For this review, take the finished solid that the model builds, in its own axes (mm). A direction names the side the tool comes from. Coordinates: 2 decimals unless noted, no trailing zeros. Loops run counter-clockwise (first coordinate to the right, second up) from the corner with the lowest first, then second, coordinate; pieces in that order, holes last. Notation, with made-up numbers: M 66,61 L 107,61 A17 cw 107,83 Z; hole C 30.5,-34 d9. An arc over 180 degrees is marked long. Use one line per item in the form item = value.
```python
from build123d import *

# Parameters (mm, degrees)
F0_W     = 80
F0_H     = 40
F1_DEPTH = 10
F2_W     = 74
F2_H     = 26
F3_DEPTH = 5
F4_W     = 4
F4_H     = 4
F5_DEPTH = 25.4
F6_W     = 4
F6_H     = 4
F7_DEPTH = 50.8


with BuildPart() as f1:
    # F0 (on Front) → F1 (new body)
    with BuildSketch(Plane.XZ):
        with Locations((40, 20)):
            Rectangle(F0_W, F0_H)
    extrude(amount=F1_DEPTH)

    # F2 (on face) → F3 (cut)
    with BuildSketch(Plane.XZ.offset(10)):
        with Locations((40, 20)):
            Rectangle(F2_W, F2_H)
    extrude(amount=-F3_DEPTH, mode=Mode.SUBTRACT)

    # F4 (on face) → F5 (cut)
    with BuildSketch(Plane.XZ.offset(10)):
        with Locations((6, 38)):
            Rectangle(F4_W, F4_H)
        with Locations((74, 38)):
            Rectangle(F4_W, F4_H)
        with Locations((74, 2)):
            Rectangle(F4_W, F4_H)
        with Locations((6, 2)):
            Rectangle(F4_W, F4_H)
    extrude(amount=-F5_DEPTH, mode=Mode.SUBTRACT)

    # F6 (on face) → F7 (cut)
    with BuildSketch(Plane.XY.offset(40)):
        with Locations((6, -2)):
            Rectangle(F6_W, F6_H)
        with Locations((74, -2)):
            Rectangle(F6_W, F6_H)
    extrude(amount=-F7_DEPTH, mode=Mode.SUBTRACT)


solid = f1.part
```
1. Draft analysis for pull direction Z (two halves, no side actions). For faces 1 (the face through (39, -8, 7)), 2 (the face through (74, -7, 4)), 3 (the face through (6, -4, 20)), 4 (the face through (39, -8, 33)), state which applies: +Z half, -Z half, draft (parallel to the pull), parting line (faces both ways), or undercut.
Computed values:
face_1 = undercut
face_2 = -Z half
face_3 = draft
face_4 = undercut
2. For pin 1 Ø1.2 at (x, y) = (74.5, -7) entering from -Z; pin 2 Ø1 at (x, z) = (13, 13.5) entering from -Y; pin 3 Ø1.2 at (x, z) = (5.5, 26.5) entering from +Y, all flat-tipped, find the tip position at first contact; note any pin that passes through.
Computed values:
pin_1 = 4
pin_2 = -5
pin_3 = -4
3. Consider section D-D on y = -8.5. Write out the cut boundary in (x, z).
Computed values:
outline = M 0,0 L 4,0 L 4,4 L 8,4 L 8,0 L 72,0 L 72,4 L 76,4 L 76,0 L 80,0 L 80,40 L 76,40 L 76,36 L 72,36 L 72,40 L 8,40 L 8,36 L 4,36 L 4,40 L 0,40 Z; hole M 3,7 L 77,7 L 77,33 L 3,33 Z
4. Consider section B-B on x = 7. Write out the cut boundary in (y, z).
Computed values:
outline = M -10,4 L -4,4 L -4,36 L -10,36 L -10,33 L -5,33 L -5,7 L -10,7 Z
5. Consider section C-C on z = 34.5. Write out the cut boundary in (x, y).
Computed values:
outline = M 0,-10 L 80,-10 L 80,0 L 76,0 L 76,-4 L 72,-4 L 72,0 L 8,0 L 8,-4 L 4,-4 L 4,0 L 0,0 Z
6. Tool access review of faces 5 (the face through (6, -7, 4)), 6 (the face through (74, -7, 36)), 7 (the face through (39, -5, 20)): name each direction out of +Z, -Z, +X, -X, +Y, -Y from which nothing blocks a thin tool from reaching the whole face with its end or side.
Computed values:
face_5 = -Z, +Y, -Y
face_6 = +Z, +Y, -Y
face_7 = -Y
7. Consider section A-A on y = -1.5. Write out the cut boundary in (x, z).
Computed values:
outline = M 0,0 L 4,0 L 4,40 L 0,40 Z; M 8,0 L 72,0 L 72,40 L 8,40 Z; M 76,0 L 80,0 L 80,40 L 76,40 Z
8. Wall thickness on line 1 along X through (y, z) = (-3.75, 10); line 2 along Z through (x, y) = (53, -9); line 3 along Z through (x, y) = (6.5, -6.25): over which ranges is each line inside the solid? List them lowest first. Write a range as from..to.
Computed values:
line_1 = 0..4, 8..72, 76..80
line_2 = 0..7, 33..40
line_3 = 4..7, 33..36
